```python
from build123d import *

# Parameters (mm, degrees)
SKETCH1_W           = 40.4
SKETCH1_H           = 35
SKETCH1_R           = 2
BOSS_EXTRUDE1_DEPTH = 15
SKETCH2_R           = 2
BOSS_EXTRUDE2_DEPTH = 1.5
SKETCH3_R           = 4
CUT_EXTRUDE1_DEPTH  = 15
SKETCH4_W           = 13
SKETCH4_H           = 3.8
SKETCH4_W_2         = 3
SKETCH4_H_2         = 3
SKETCH4_W_3         = 18.15
SKETCH4_W_4         = 2.5
SKETCH4_H_3         = 2
BOSS_EXTRUDE3_DEPTH = 1.1
SKETCH5_W           = 3
SKETCH5_H           = 3.5
SKETCH5_W_2         = 2.5
SKETCH5_H_2         = 2.5
SKETCH5_H_3         = 4.3
BOSS_EXTRUDE4_DEPTH = 1
CHAMFER1_SIZE       = 0.5
CUT_EXTRUDE2_REACH  = 9.318
SKETCH6_W           = 8.5
SKETCH6_H           = 3.5
CHAMFER2_SIZE       = 0.8
FILLET1_R           = 2
CUT_EXTRUDE3_REACH  = 3.5
SKETCH7_R           = 1.5


with BuildPart() as part:
    # Sketch1 → Boss-Extrude1 (new body)
    with BuildSketch(Plane(origin=(0, 0, 0), x_dir=(1, 0, 0), z_dir=(0, 1, 0))):
        with BuildLine():
            Line((-21.7, 15.817500063), (-21.7, -15.817500063))
            Line((-21.7, -15.817500063), (-23.204723756, -15.817500063))
            ThreePointArc((-23.204723756, -15.817500063), (-26.386704272, -23.499480579), (-18.704723756, -20.317500063))
            Line((-18.704723756, -20.317500063), (-18.704723756, -19))
            Line((-18.704723756, -19), (18.704723756, -19))
            Line((18.704723756, -19), (18.704723756, -20.317500063))
            ThreePointArc((18.704723756, -20.317500063), (26.386704272, -23.499480579), (23.204723756, -15.817500063))
            Line((23.204723756, -15.817500063), (21.7, -15.817500063))
            Line((21.7, -15.817500063), (21.7, 15.817500063))
            Line((21.7, 15.817500063), (23.204723756, 15.817500063))
            ThreePointArc((23.204723756, 15.817500063), (26.386704272, 23.499480579), (18.704723756, 20.317500063))
            Line((18.704723756, 20.317500063), (18.704723756, 19))
            Line((18.704723756, 19), (-18.704723756, 19))
            Line((-18.704723756, 19), (-18.704723756, 20.317500063))
            ThreePointArc((-18.704723756, 20.317500063), (-26.386704272, 23.499480579), (-23.204723756, 15.817500063))
            Line((-23.204723756, 15.817500063), (-21.7, 15.817500063))
        make_face()
        Rectangle(SKETCH1_W, SKETCH1_H, mode=Mode.SUBTRACT)
        with Locations((-23.204723756, 20.317500063)):
            Circle(SKETCH1_R, mode=Mode.SUBTRACT)
        with Locations((-23.204723756, -20.317500063)):
            Circle(SKETCH1_R, mode=Mode.SUBTRACT)
        with Locations((23.204723756, 20.317500063)):
            Circle(SKETCH1_R, mode=Mode.SUBTRACT)
        with Locations((23.204723756, -20.317500063)):
            Circle(SKETCH1_R, mode=Mode.SUBTRACT)
    extrude(amount=BOSS_EXTRUDE1_DEPTH)

    # Sketch2 → Boss-Extrude2 (add)
    with BuildSketch(Plane(origin=(0, 15, 0), x_dir=(1, 0, 0), z_dir=(0, 1, 0))):
        with BuildLine():
            Line((-21.7, 15.817500063), (-21.7, -15.817500063))
            Line((-21.7, -15.817500063), (-23.204723756, -15.817500063))
            ThreePointArc((-23.204723756, -15.817500063), (-26.386704272, -23.499480579), (-18.704723756, -20.317500063))
            Line((-18.704723756, -20.317500063), (-18.704723756, -19))
            Line((-18.704723756, -19), (18.704723756, -19))
            Line((18.704723756, -19), (18.704723756, -20.317500063))
            ThreePointArc((18.704723756, -20.317500063), (26.386704272, -23.499480579), (23.204723756, -15.817500063))
            Line((23.204723756, -15.817500063), (21.7, -15.817500063))
            Line((21.7, -15.817500063), (21.7, 15.817500063))
            Line((21.7, 15.817500063), (23.204723756, 15.817500063))
            ThreePointArc((23.204723756, 15.817500063), (26.386704272, 23.499480579), (18.704723756, 20.317500063))
            Line((18.704723756, 20.317500063), (18.704723756, 19))
            Line((18.704723756, 19), (-18.704723756, 19))
            Line((-18.704723756, 19), (-18.704723756, 20.317500063))
            ThreePointArc((-18.704723756, 20.317500063), (-26.386704272, 23.499480579), (-23.204723756, 15.817500063))
            Line((-23.204723756, 15.817500063), (-21.7, 15.817500063))
        make_face()
        with Locations((23.204723756, -20.317500063)):
            Circle(SKETCH2_R, mode=Mode.SUBTRACT)
        with Locations((23.204723756, 20.317500063)):
            Circle(SKETCH2_R, mode=Mode.SUBTRACT)
        with Locations((-23.204723756, 20.317500063)):
            Circle(SKETCH2_R, mode=Mode.SUBTRACT)
        with Locations((-23.204723756, -20.317500063)):
            Circle(SKETCH2_R, mode=Mode.SUBTRACT)
    extrude(amount=BOSS_EXTRUDE2_DEPTH)

    # Sketch3 → Cut-Extrude1 (cut)
    with BuildSketch(Plane(origin=(0, 16.5, 0), x_dir=(1, 0, 0), z_dir=(0, 1, 0))):
        with Locations((-23.204723756, -20.317500063)):
            Circle(SKETCH3_R)
        with Locations((-23.204723756, 20.317500063)):
            Circle(SKETCH3_R)
        with Locations((23.204723756, 20.317500063)):
            Circle(SKETCH3_R)
        with Locations((23.204723756, -20.317500063)):
            Circle(SKETCH3_R)
    extrude(amount=-CUT_EXTRUDE1_DEPTH, mode=Mode.SUBTRACT)

    # Sketch4 → Boss-Extrude3 (add)
    with BuildSketch(Plane.XZ.offset(-15)):
        with Locations((-13.7, 15.6)):
            Rectangle(SKETCH4_W, SKETCH4_H)
        with Locations((-18.7, -16)):
            Rectangle(SKETCH4_W_2, SKETCH4_H_2)
        with Locations((11.125, 15.6)):
            Rectangle(SKETCH4_W_3, SKETCH4_H)
        with Locations((13.2, -16.5)):
            Rectangle(SKETCH4_W_4, SKETCH4_H_3)
    extrude(amount=BOSS_EXTRUDE3_DEPTH)

    # Sketch5 → Boss-Extrude4 (add)
    with BuildSketch(Plane.XZ.offset(-13.9)):
        with Locations((-18.7, -15.75)):
            Rectangle(SKETCH5_W, SKETCH5_H)
        with Locations((13.2, -16.25)):
            Rectangle(SKETCH5_W_2, SKETCH5_H_2)
        with Locations((-13.7, 15.35)):
            Rectangle(SKETCH5_W, SKETCH5_H_3)
        with Locations((11.125, 15.35)):
            Rectangle(SKETCH5_W, SKETCH5_H_3)
    extrude(amount=BOSS_EXTRUDE4_DEPTH)

    # Chamfer1
    chamfer1_edges = [part.edges().sort_by_distance(p)[0] for p in [
        (-18.7, 12.9, -14),
        (13.2, 12.9, -15),
    ]]
    chamfer(chamfer1_edges, length=CHAMFER1_SIZE)

    # Sketch6 → Cut-Extrude2 (cut, up to next)
    with BuildSketch(Plane(origin=(0, 0, 17.5), x_dir=(-1, 0, 0), z_dir=(0, 0, -1)), mode=Mode.PRIVATE) as cut_extrude2_sk1:
        with Locations((2.575, 12.8)):
            Rectangle(SKETCH6_W, SKETCH6_H)
    cut_extrude2_tool1 = extrude(cut_extrude2_sk1.sketch, amount=-CUT_EXTRUDE2_REACH, mode=Mode.PRIVATE) & part.part
    add(cut_extrude2_tool1.solids().sort_by_distance((-2.575, 12.8, 17.5))[0], mode=Mode.SUBTRACT)

    # Chamfer2
    chamfer2_edges = [part.edges().sort_by_distance(p)[0] for p in [
        (-6.825, 14.55, 18.25),
        (1.675, 14.55, 18.25),
    ]]
    chamfer(chamfer2_edges, length=CHAMFER2_SIZE)

    # Fillet1
    fillet1_edges = [part.edges().sort_by_distance(p)[0] for p in [
        (-20.2, 6.95, 17.5),
        (20.2, 6.95, 17.5),
        (-20.2, 6.45, -17.5),
        (20.2, 7.5, -17.5),
    ]]
    fillet(fillet1_edges, radius=FILLET1_R)

    # Sketch7 → Cut-Extrude3 (cut, up to next)
    with BuildSketch(Plane.XZ.offset(-15), mode=Mode.PRIVATE) as cut_extrude3_sk1:
        with Locations((0, -12.5)):
            Circle(SKETCH7_R)
    cut_extrude3_tool1 = extrude(cut_extrude3_sk1.sketch, amount=-CUT_EXTRUDE3_REACH, mode=Mode.PRIVATE) & part.part
    add(cut_extrude3_tool1.solids().sort_by_distance((0, 15, -12.5))[0], mode=Mode.SUBTRACT)


solid = part.part
```
The model under review builds one solid part; all positions refer to its coordinate system, in mm. A direction names the side the tool comes from. Round coordinates to 2 decimals unless told otherwise and drop trailing zeros. Loops run counter-clockwise (first coordinate to the right, second up) from the corner with the lowest first, then second, coordinate; pieces in that order, holes last. Notation, with made-up numbers: (76, 72) - (100, 72) arc R23 ccw to (100, 94) - close; hole circle Ø4 at (35, 48.25). An arc over 180 degrees is marked (long way). Use a Markdown table: item, result. Add a question column.
Q1. Add section C-C (y = 6). State the section outline as (x, z) points, plus the area to 3 significant figures.
Q2. Add section D-D (z = 4.5). State the section outline as (x, y) points.
Q3. For probe 1 along X at (y, z) = (14.5, 10); probe 2 along Z at (x, y) = (15, 8.5); probe 3 along Z at (x, y) = (20.5, 15.75), list the stretches that pass through material, from the lowest coordinate up.
Q4. Add section A-A (z = -12.5). State the section outline as (x, y) points.
Q5. Insertion check: pin 1 Ø12 at (x, z) = (-7.5, 12.5) entering from -Y; pin 2 Ø1 at (x, y) = (1, 12.5) entering from +Z; pin 3 Ø2 at (y, z) = (7, 6.5) entering from +X; pin 4 Ø1.5 at (x, z) = (3.5, -5.5) entering from -Y. Each pin has a flat end and moves straight along its axis. Give the tip position at first contact, or say it passes through.
Q6. The part is to be moulded in two halves that separate along X. For faces 1 (the face through (21.7, 8, 0)), 2 (the face through (18.705, 8, -20)), say which applies: pulls with the +X half, pulls with the -X half, needs draft (parallel to the pull), parting line crosses it, or undercut.
Q7. Machinability: for faces 3 (the face through (-25, 1.5, -19)), 4 (the face through (0, 8, 19)), 5 (the face through (14.45, 14, -17)), which of the approach directions +Z, -Z, +X, -X, +Y, -Y give a long, thin tool a straight path to every point of the face, cutting with its end or side? Answer none if there is none.
Q8. Add section B-B (x = 3). State the section outline as (y, z) points, plus the area to 3 significant figures.
Worked answers:
| question | item | result |
|---|---|---|
| 1 | outline | (-23.2, -15.82) arc R4.5 ccw (long way) to (-18.7, -20.32) - (-18.7, -19) - (18.7, -19) - (18.7, -20.32) arc R4.5 ccw (long way) to (23.2, -15.82) - (21.7, -15.82) - (21.7, 15.82) - (23.2, 15.82) arc R4.5 ccw (long way) to (18.7, 20.32) - (18.7, 19) - (-18.7, 19) - (-18.7, 20.32) arc R4.5 ccw (long way) to (-23.2, 15.82) - (-21.7, 15.82) - (-21.7, -15.82) - close; hole circle Ø8 at (-23.2, -20.32); hole circle Ø8 at (-23.2, 20.32); hole (-20.2, -15.5) arc R2 ccw to (-18.2, -17.5) - (18.2, -17.5) arc R2 ccw to (20.2, -15.5) - (20.2, 15.5) arc R2 ccw to (18.2, 17.5) - (-18.2, 17.5) arc R2 ccw to (-20.2, 15.5) - close; hole circle Ø8 at (23.2, -20.32); hole circle Ø8 at (23.2, 20.32) |
| 1 | area | 271 mm² |
| 2 | outline | (-21.7, 0) - (-20.2, 0) - (-20.2, 15) - (20.2, 15) - (20.2, 0) - (21.7, 0) - (21.7, 16.5) - (-21.7, 16.5) - close |
| 3 | probe 1 | -21.7 to -20.2, 20.2 to 21.7 |
| 3 | probe 2 | -19 to -17.5, 17.5 to 19 |
| 3 | probe 3 | -23.91 to -23.26, -17.37 to 17.37, 23.26 to 23.91 |
| 4 | outline | (-21.7, 0) - (-20.2, 0) - (-20.2, 15) - (-1.5, 15) - (-1.5, 16.5) - (-21.7, 16.5) - close; (1.5, 15) - (20.2, 15) - (20.2, 0) - (21.7, 0) - (21.7, 16.5) - (1.5, 16.5) - close |
| 5 | pin 1 | y = 0 |
| 5 | pin 2 | z = -17.5 |
| 5 | pin 3 | x = 21.7 |
| 5 | pin 4 | y = 15 |
| 6 | face 1 | pulls with the +X half |
| 6 | face 2 | undercut |
| 7 | face 3 | +Y |
| 7 | face 4 | +Z, +Y, -Y |
| 7 | face 5 | -Y |
| 8 | outline | (0, -19) - (16.5, -19) - (16.5, 19) - (0, 19) - (0, 17.5) - (13.9, 17.5) - (13.9, 13.7) - (15, 13.7) - (15, -17.5) - (0, -17.5) - close |
| 8 | area | 106 mm² |
